Verification items for the finished model (mm, model axes). A direction names the side the tool comes from. Coordinates: 2 decimals unless noted, no trailing zeros. Order: outer loops, then holes, each group sorted by start corner. A loop starts at its lowest first (then second) coordinate and runs counter-clockwise, first axis right, second up. Notation, with made-up numbers: M 3.5,-1.5 L 38.5,-1.5 A28 ccw 38.5,22.5 Z; hole C 35,-38.5 d1. An arc over 180 degrees is marked long. Return JSON: item names as keys, results as strings. Group by question number.
Q1. Section check C-C, the plane x = 89. Enter the section's corners in (y, z).
Q2. Mould release check, pull along Z, two halves, no side actions. Record for faces 1 (the face through (76.94, 3, -59)), 2 (the face through (3, 3, -16.486)), 3 (the face through (201, 3, -66.2)): pulls with the +Z half, pulls with the -Z half, needs draft (parallel to the pull), parting line crosses it, or undercut.
Q3. Section check B-B, the plane x = 23.5. Enter the section's corners in (y, z), then the cut area to 3 significant figures.
Q4. Access from +Z, -Z, +X, -X, +Y, -Y to the whole of each face (thin tool, end or side, straight path). Record for faces 4 (the face through (6.35, 3, -37)), 5 (the face through (21.06, 3, -59)), 6 (the face through (26.14, 3, -59)), 7 (the face through (128.571, 3, -3)).
Q5. Go/stop test with flat-tipped pins: pin 1 Ø1.9 at (y, z) = (1.5, -4) entering from +X; pin 2 Ø3 at (x, y) = (208.5, 2) entering from -Z; pin 3 Ø1.9 at (x, y) = (88, 4) entering from +Z. Record where each tip stops, or that it passes through.
Q6. Section check A-A, the plane z = -4. Enter the section's corners in (x, y).
Q7. Thickness scan on probe 1 along X at (y, z) = (6, -62); probe 2 along X at (y, z) = (4.75, -41.5); probe 3 along X at (y, z) = (5, -37). Record the ranges inside material, lowest first.
from build123d import *

# Parameters (mm, degrees)
SKETCH1_W           = 32.142857142
SKETCH1_H           = 6.35
SKETCH1_W_2         = 32.142857143
SKETCH1_W_3         = 6.35
SKETCH1_H_2         = 8.242857143
SKETCH1_H_3         = 8.242857142
BOSS_EXTRUDE1_DEPTH = 6.35
SKETCH2_W           = 212.3
SKETCH2_H           = 6.35
SKETCH2_W_2         = 5.08
SKETCH2_H_2         = 8.5
BOSS_EXTRUDE2_DEPTH = 6.35
SKETCH3_W           = 35
SKETCH3_H           = 26
CUT_EXTRUDE1_DEPTH  = 235.622595885
SKETCH4_W           = 14.71
SKETCH4_H           = 6.35
SKETCH4_W_2         = 20.32
CUT_EXTRUDE2_DEPTH  = 6.35
SKETCH5_W           = 20.32
SKETCH5_H           = 6.35
SKETCH5_W_2         = 18.06
CUT_EXTRUDE3_DEPTH  = 235.622595885
SKETCH8_W           = 15
SKETCH8_H           = 12.5
CUT_EXTRUDE6_DEPTH  = 235.622595885


with BuildPart() as part:
    # Sketch1 → Boss-Extrude1 (new body)
    with BuildSketch(Plane(origin=(0, 0, 0), x_dir=(1, 0, 0), z_dir=(0, 1, 0))):
        Polygon((6.35, 6.35), (32.142857143, 6.35), (64.285714286, 6.35), (96.428571429, 6.35), (128.571428571, 6.35), (160.714285714, 6.35), (192.857142857, 6.35), (218.65, 6.35), (218.65, 8.242857143), (218.65, 16.485714286), (218.65, 24.728571429), (218.65, 32.971428571), (218.65, 41.214285714), (218.65, 49.457142857), (218.65, 51.35), (192.857142857, 51.35), (160.714285714, 51.35), (128.571428571, 51.35), (96.428571429, 51.35), (64.285714286, 51.35), (32.142857143, 51.35), (6.35, 51.35), (6.35, 49.457142857), (6.35, 41.214285714), (6.35, 32.971428571), (6.35, 24.728571429), (6.35, 16.485714286), (6.35, 8.242857143), align=None)
        with Locations((112.5, 54.525)):
            Rectangle(SKETCH1_W, SKETCH1_H)
        with Locations((112.5, 3.175)):
            Rectangle(SKETCH1_W, SKETCH1_H)
        with Locations((176.785714286, 3.175)):
            Rectangle(SKETCH1_W_2, SKETCH1_H)
        with Locations((176.785714286, 54.525)):
            Rectangle(SKETCH1_W_2, SKETCH1_H)
        with Locations((48.214285715, 54.525)):
            Rectangle(SKETCH1_W_2, SKETCH1_H)
        with Locations((48.214285715, 3.175)):
            Rectangle(SKETCH1_W_2, SKETCH1_H)
        with Locations((3.175, 12.364285714)):
            Rectangle(SKETCH1_W_3, SKETCH1_H_2)
        with Locations((3.175, 28.85)):
            Rectangle(SKETCH1_W_3, SKETCH1_H_3)
        with Locations((3.175, 45.335714286)):
            Rectangle(SKETCH1_W_3, SKETCH1_H_2)
        with Locations((221.825, 12.364285714)):
            Rectangle(SKETCH1_W_3, SKETCH1_H_2)
        with Locations((221.825, 28.85)):
            Rectangle(SKETCH1_W_3, SKETCH1_H_3)
        with Locations((221.825, 45.335714286)):
            Rectangle(SKETCH1_W_3, SKETCH1_H_2)
    extrude(amount=BOSS_EXTRUDE1_DEPTH)

    # Sketch2 → Boss-Extrude2 (add)
    with BuildSketch(Plane(origin=(0, 6.35, 0), x_dir=(1, 0, 0), z_dir=(0, 1, 0))):
        with Locations((112.5, 54.525)):
            Rectangle(SKETCH2_W, SKETCH2_H)
        with Locations((23.6, 61.95)):
            Rectangle(SKETCH2_W_2, SKETCH2_H_2)
        with Locations((49, 61.95)):
            Rectangle(SKETCH2_W_2, SKETCH2_H_2)
        with Locations((74.4, 61.95)):
            Rectangle(SKETCH2_W_2, SKETCH2_H_2)
        with Locations((99.8, 61.95)):
            Rectangle(SKETCH2_W_2, SKETCH2_H_2)
        with Locations((201.4, 61.95)):
            Rectangle(SKETCH2_W_2, SKETCH2_H_2)
        with Locations((176, 61.95)):
            Rectangle(SKETCH2_W_2, SKETCH2_H_2)
        with Locations((125.2, 61.95)):
            Rectangle(SKETCH2_W_2, SKETCH2_H_2)
        with Locations((150.6, 61.95)):
            Rectangle(SKETCH2_W_2, SKETCH2_H_2)
    extrude(amount=-BOSS_EXTRUDE2_DEPTH)

    # Sketch3 → Cut-Extrude1 (cut, through all)
    with BuildSketch(Plane(origin=(0, 6.35, 0), x_dir=(1, 0, 0), z_dir=(0, 1, 0))):
        with Locations((112.5, 53.2)):
            Rectangle(SKETCH3_W, SKETCH3_H)
    extrude(amount=-CUT_EXTRUDE1_DEPTH, mode=Mode.SUBTRACT)

    # Sketch4 → Cut-Extrude2 (cut)
    with BuildSketch(Plane(origin=(0, 6.35, 0), x_dir=(1, 0, 0), z_dir=(0, 1, 0))):
        with Locations((13.705, 54.525)):
            Rectangle(SKETCH4_W, SKETCH4_H)
        with Locations((36.3, 54.525)):
            Rectangle(SKETCH4_W_2, SKETCH4_H)
        with Locations((211.295, 54.525)):
            Rectangle(SKETCH4_W, SKETCH4_H)
        with Locations((188.7, 54.525)):
            Rectangle(SKETCH4_W_2, SKETCH4_H)
    extrude(amount=-CUT_EXTRUDE2_DEPTH, mode=Mode.SUBTRACT)

    # Sketch5 → Cut-Extrude3 (cut, through all)
    with BuildSketch(Plane(origin=(0, 6.35, 0), x_dir=(1, 0, 0), z_dir=(0, 1, 0))):
        with Locations((61.7, 54.525)):
            Rectangle(SKETCH5_W, SKETCH5_H)
        with Locations((85.97, 54.525)):
            Rectangle(SKETCH5_W_2, SKETCH5_H)
        with Locations((139.03, 54.525)):
            Rectangle(SKETCH5_W_2, SKETCH5_H)
        with Locations((163.3, 54.525)):
            Rectangle(SKETCH5_W, SKETCH5_H)
    extrude(amount=-CUT_EXTRUDE3_DEPTH, mode=Mode.SUBTRACT)

    # Sketch8 → Cut-Extrude6 (cut, through all)
    with BuildSketch(Plane(origin=(0, 6.35, 0), x_dir=(1, 0, 0), z_dir=(0, 1, 0))):
        with Locations((176, 37.15)):
            Rectangle(SKETCH8_W, SKETCH8_H)
    extrude(amount=-CUT_EXTRUDE6_DEPTH, mode=Mode.SUBTRACT)


solid = part.part
Numbers:
{
 "1": {"outline": "M 0,-51.35 L 6.35,-51.35 L 6.35,-6.35 L 0,-6.35 Z"},
 "2": {"face 1": "needs draft", "face 2": "undercut", "face 3": "pulls with the -Z half"},
 "3": {"outline": "M 0,-66.2 L 6.35,-66.2 L 6.35,-6.35 L 0,-6.35 Z", "area": "380 mm2"},
 "4": {"face 4": "-X, +Y, -Y", "face 5": "-Z, -X, +Y, -Y", "face 6": "-Z, +Y, -Y", "face 7": "+Z, +Y, -Y"},
 "5": {"pin 1": "stops at x = 192.86", "pin 2": "stops at z = -51.35", "pin 3": "stops at z = -6.35"},
 "6": {"outline": "M 32.14,0 L 64.29,0 L 64.29,6.35 L 32.14,6.35 Z; M 96.43,0 L 128.57,0 L 128.57,6.35 L 96.43,6.35 Z; M 160.71,0 L 192.86,0 L 192.86,6.35 L 160.71,6.35 Z"},
 "7": {"probe 1": "x = 21.06 to 26.14, 46.46 to 51.54, 71.86 to 76.94, 148.06 to 153.14, 173.46 to 178.54, 198.86 to 203.94", "probe 2": "x = 0 to 95, 130 to 168.5, 183.5 to 225", "probe 3": "x = 6.35 to 168.5, 183.5 to 218.65"}
}
